Source: CAD feature listing. Evaluate the final solid. Frame: model axes, mm. Face numbers are marked on the shaded views. A direction names the side the tool comes from. Round coordinates to 2 decimals unless told otherwise and drop trailing zeros. Order: outer loops, then holes, each group sorted by start corner. A loop starts at its lowest first (then second) coordinate and runs counter-clockwise, first axis right, second up. Notation, with made-up numbers: (21.25, 45.5) - (79.25, 45.5) arc R32 cw to (79.25, 83.5) - close; hole circle Ø3 at (18.25, 51.5). An arc over 180 degrees is marked (long way). Use one line per item in the form item = value. Start each with the question number.
Q1. Set-up query: the marked faces 1, 2 and 3. Return all of +Z, -Z, +X, -X, +Y, -Y with unobstructed straight access to the full face (end or side cutting, diameter ignored); none if empty.
Q2. Pin query (flat end, axial travel): pin 1 Ø3 at (y, z) = (128.5, 86) entering from +X; pin 2 Ø6 at (x, z) = (-27.5, 176) entering from +Y; pin 3 Ø3 at (y, z) = (93.5, 128.5) entering from -X. Return the tip coordinate at first contact, or that it passes through.
Q3. Cut plane C-C, the plane x = 27. Return the cut outline in (y, z), and give its area (3 significant figures).
Q4. Draft query along X for the marked faces 4, 5 and 6. Return one class per face: released by +X, released by -X, zero draft, split by the parting line, or undercut.
Q5. Cut plane B-B, the plane z = 226.5. Return the cut outline in (x, y).
Q6. Cut plane A-A, the plane y = -129. Return the cut outline in (x, z).
Q7. Ray query, line 1 (Y direction, x = 165, z = 84); line 2 (X direction, y = 55, z = 84); line 3 (X direction, y = -107, z = 56). Return the intervals inside material, ascending. Write a range as [from, to].
Q8. Cut plane D-D, the plane y = 134. Return the cut outline in (x, z).
from build123d import *

# Parameters (mm, degrees)
F1_DEPTH = 299.72


with BuildPart() as f1:
    # F0 (on Top) → F1 (new body)
    with BuildSketch(Plane.XY):
        with BuildLine():
            Line((-111.383964, 50.262654), (-283.667104, 50.262654))
            Line((-283.667104, 50.262654), (-283.667104, -89.717354))
            Line((-283.667104, -89.717354), (-239.49016, -89.717354))
            ThreePointArc((-239.49016, -89.717354), (-175.99016, -26.217354), (-112.49016, -89.717354))
            Line((-112.49016, -89.717354), (166.092987, -89.717354))
            ThreePointArc((166.092987, -89.717354), (229.592987, -26.217354), (293.092987, -89.717354))
            ThreePointArc((293.092987, -89.717354), (293.092302, -90.012305), (293.090247, -90.30725))
            Line((293.090247, -90.30725), (340.859073, -89.717354))
            Line((340.859073, -89.717354), (340.859073, 50.262654))
            Line((340.859073, 50.262654), (164.986756, 179.474962))
            Line((164.986756, 179.474962), (10.649873, 179.474962))
            Line((10.649873, 179.474962), (-111.383964, 50.262654))
        make_face()
        with BuildLine():
            ThreePointArc((-112.49016, -89.717354), (-175.99016, -26.217354), (-239.49016, -89.717354))
            ThreePointArc((-239.49016, -89.717354), (-175.99016, -153.217354), (-112.49016, -89.717354))
        make_face()
        with BuildLine():
            ThreePointArc((293.092987, -89.717354), (229.592987, -26.217354), (166.092987, -89.717354))
            ThreePointArc((166.092987, -89.717354), (229.298036, -153.216669), (293.090247, -90.30725))
            ThreePointArc((293.090247, -90.30725), (293.092302, -90.012305), (293.092987, -89.717354))
        make_face()
    extrude(amount=F1_DEPTH)


solid = f1.part
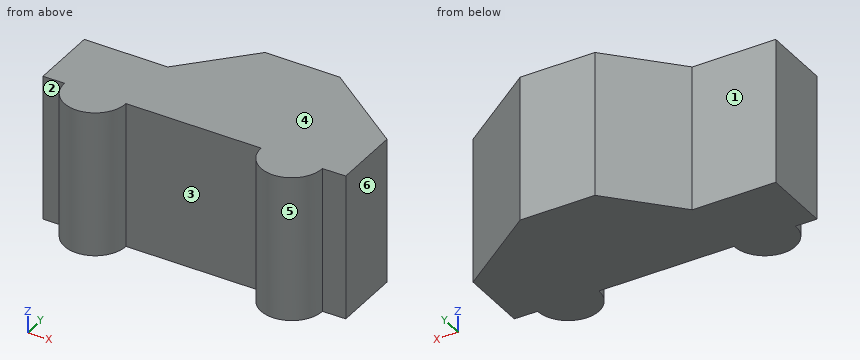
Completed:
q1.face_1 = +Z, -Z, -X, +Y
q1.face_2 = +Z, -Z, -X, -Y
q1.face_3 = +Z, -Z, -Y
q2.pin_1 = 236.41
q2.pin_2 = 142.26
q2.pin_3 = -71.97
q3.outline = (-89.72, 0) - (179.47, 0) - (179.47, 299.72) - (-89.72, 299.72) - close
q3.area = 80,700 mm2
q4.face_4 = zero draft
q4.face_5 = undercut
q4.face_6 = released by +X
q5.outline = (-283.67, -89.72) - (-239.49, -89.72) arc R63.5 ccw to (-112.49, -89.72) - (166.09, -89.72) arc R63.5 ccw to (293.09, -90.31) - (340.86, -89.72) - (340.86, 50.26) - (164.99, 179.47) - (10.65, 179.47) - (-111.38, 50.26) - (-283.67, 50.26) - close
q6.outline = (-225.88, 0) - (-126.1, 0) - (-126.1, 299.72) - (-225.88, 299.72) - close; (179.7, 0) - (279.48, 0) - (279.48, 299.72) - (179.7, 299.72) - close
q7.line_1 = [-89.72, 179.47]
q7.line_2 = [-106.91, 334.41]
q7.line_3 = [-237.09, -114.89], [168.49, 290.7]
q8.outline = (-32.3, 0) - (226.88, 0) - (226.88, 299.72) - (-32.3, 299.72) - close
